CAD build for the part. Positions are in the model's coordinates, mm. Face numbers are marked on the shaded views. A direction names the side the tool comes from. Round coordinates to 2 decimals unless told otherwise and drop trailing zeros. Write each loop counter-clockwise with the first axis right and the second up, starting at its lowest first coordinate (ties: lowest second). Pieces come first, ordered by that corner, then holes. Notation, with made-up numbers: (64, -23.75) - (82, -23.75) arc R11 ccw to (82, -7.75) - close; hole circle Ø7 at (-22.5, -3). An arc over 180 degrees is marked (long way). Use one line per item in the form item = value. Start each with the question number.
Item 1: Pull direction Y, two halves, no side cores. Call the marked faces 4, 5 and 6: +Y half, -Y half, draft (parallel to the pull), parting line (faces both ways), or undercut.
Item 2: Band-saw the part on B-B, the plane x = 23.5. List the corners of the cut face in (y, z), and give its area (3 significant figures).
Item 3: Drill centre lines: L1, parallel to Y at x = 0, z = -13.5; L2, parallel to Y at x = 0, z = 15.5; L3, parallel to X at y = 14.5, z = 3. Where is each one in solid material? Low to high.
Item 4: Tool access for the marked faces 1, 2 and 3: list every direction of +Z, -Z, +X, -X, +Y, -Y with a clear straight run to the whole face (end or side of a thin tool).
Item 5: Band-saw the part on D-D, the plane z = 13.5. List the corners of the cut face in (x, y), and give its area (3 significant figures).
Item 6: Band-saw the part on A-A, the plane z = -23.5. List the corners of the cut face in (x, y).
Item 7: Band-saw the part on C-C, the plane y = 0. Give the number of separate pieces and of enclosed holes in the cut face, and give its area (3 significant figures).
Item 8: Pin check, flat tips, straight feed: pin 1 (3 mm diameter, centred on y = -0.5, z = -44, fed in from -X); pin 2 (5 mm diameter, centred on x = -3.5, y = -9.5, fed in from -Z); pin 3 (6 mm diameter, centred on x = 12, y = -34, fed in from +Z). Stop position of each tip, or through.
from build123d import *

# Parameters (mm, degrees)
SKETCH1_R           = 7.5
BOSS_EXTRUDE1_DEPTH = 32.5
SKETCH3_R           = 5
BOSS_EXTRUDE3_DEPTH = 48.5
SKETCH4_R           = 54
SKETCH4_R_2         = 35
BOSS_EXTRUDE4_DEPTH = 25
SKETCH5_R           = 15
SKETCH5_W           = 8
SKETCH5_H           = 20.543167705
BOSS_EXTRUDE5_DEPTH = 5
SKETCH6_R           = 10
BOSS_EXTRUDE6_DEPTH = 25
SKETCH7_W           = 1
SKETCH7_H           = 6
CUT_EXTRUDE1_DEPTH  = 16
CUT_EXTRUDE2_START  = -48.5
SKETCH8_R           = 3
CUT_EXTRUDE2_DEPTH  = 48.5


with BuildPart() as part:
    # Sketch1 → Boss-Extrude1 (new, symmetric)
    with BuildSketch(Plane.XY):
        Circle(SKETCH1_R)
    extrude(amount=BOSS_EXTRUDE1_DEPTH, both=True)

    # Sketch3 → Boss-Extrude3 (add, symmetric)
    with BuildSketch(Plane.XY):
        with Locations(Location((0, 0, 0), (0, 0, 180))):
            Circle(SKETCH3_R)
    extrude(amount=BOSS_EXTRUDE3_DEPTH, both=True)



with BuildPart() as body_2:
    # Sketch4 → Boss-Extrude4 (new, symmetric)
    with BuildSketch(Plane.XY):
        Circle(SKETCH4_R)
        Circle(SKETCH4_R_2, mode=Mode.SUBTRACT)
    extrude(amount=BOSS_EXTRUDE4_DEPTH, both=True)


with BuildPart() as part_1:
    add(part.part)

    add(body_2.part)  # Boss-Extrude5 merges body 2
    # Sketch5 → Boss-Extrude5 (add, symmetric)
    with BuildSketch(Plane.XY):
        Circle(SKETCH5_R)
        Polygon((14.519984026, -3.764314532), (10.519984026, -10.692517763), (28.310889132, -20.964101615), (32.310889132, -14.035898385), align=None)
        with Locations((0, 24.728416147)):
            Rectangle(SKETCH5_W, SKETCH5_H)
        Polygon((-10.519984026, -10.692517763), (-14.519984026, -3.764314532), (-32.310889132, -14.035898385), (-28.310889132, -20.964101615), align=None)
    extrude(amount=BOSS_EXTRUDE5_DEPTH, both=True)

    # Sketch6 → Boss-Extrude6 (add, symmetric)
    with BuildSketch(Plane.XY):
        Circle(SKETCH6_R)
    extrude(amount=BOSS_EXTRUDE6_DEPTH, both=True)

    # Sketch7 → Cut-Extrude1 (cut)
    with BuildSketch(Plane(origin=(0, 0, -48.5), x_dir=(-1, 0, 0), z_dir=(0, 0, -1))):
        with Locations((4.5, 0)):
            Rectangle(SKETCH7_W, SKETCH7_H)
        with Locations((-4.5, 0)):
            Rectangle(SKETCH7_W, SKETCH7_H)
    cut_extrude1 = extrude(amount=-CUT_EXTRUDE1_DEPTH, mode=Mode.SUBTRACT)

    # Mirror1: Cut-Extrude1 across plane
    add(cut_extrude1.mirror(Plane.XY), mode=Mode.SUBTRACT)

    # Sketch8 → Cut-Extrude2 (cut)
    with BuildSketch(Plane(origin=(0, 0, -48.5), x_dir=(-1, 0, 0), z_dir=(0, 0, -1)).offset(CUT_EXTRUDE2_START)):
        Circle(SKETCH8_R)
    extrude(amount=CUT_EXTRUDE2_DEPTH, mode=Mode.SUBTRACT)


solid = part_1.part
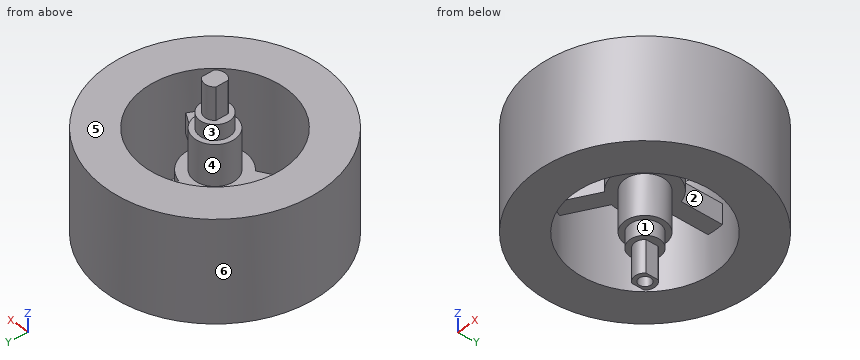
Determined:
q1.face_4 = undercut
q1.face_5 = draft
q1.face_6 = parting line
q2.outline = (-48.62, -25) - (-25.94, -25) - (-25.94, 25) - (-48.62, 25) - close; (-18.19, -5) - (-8.95, -5) - (-8.95, 5) - (-18.19, 5) - close; (25.94, -25) - (48.62, -25) - (48.62, 25) - (25.94, 25) - close
q2.area = 2,360 mm²
q3.L1 = -54 to -35, -10 to -3, 3 to 10, 35 to 54
q3.L2 = -54 to -35, -10 to 10, 35 to 54
q3.L3 = -52.02 to -31.86, -4 to 4, 31.86 to 52.02
q4.face_1 = -Z
q4.face_2 = +Z, -Z
q4.face_3 = +Z
q5.outline = circle Ø108 at (0, 0); circle Ø20 at (0, 0); hole circle Ø70 at (0, 0)
q5.area = 5,630 mm²
q6.outline = circle Ø108 at (0, 0); circle Ø20 at (0, 0); hole circle Ø70 at (0, 0); hole circle Ø6 at (0, 0)
q7.separate_pieces = 3
q7.enclosed_holes = 0
q7.area = 3,190 mm²
q8.pin_1 = -4
q8.pin_2 = -25
q8.pin_3 = 25
